Design review of the part built by this model. Coordinates are the model's own, in mm. Face numbers are marked on the shaded views. A direction names the side the tool comes from. Coordinates: 2 decimals unless noted, no trailing zeros. Loops run counter-clockwise (first coordinate to the right, second up) from the corner with the lowest first, then second, coordinate; pieces in that order, holes last. Notation, with made-up numbers: (83.5, 14.25) - (105.5, 14.25) arc R11 cw to (105.5, 34.25) - close; hole circle Ø7 at (19.5, 54). An arc over 180 degrees is marked (long way). Answer in a Markdown table with one row per item. Add a question column.
(1) Clearance check with flat-ended pins moving along their axes: pin 1 (12 mm diameter, centred on x = -8, y = 36.5, fed in from +Z); pin 2 (21 mm diameter, centred on x = 0, z = 0, fed in from -Y); pin 3 (1 mm diameter, centred on x = -13.5, y = 28.5, fed in from +Z); pin 4 (2 mm diameter, centred on y = 15.5, z = -2.5, fed in from +X). State where each tip first meets the part, or that it passes through.
(2) To check wall thickness, follow L1, parallel to Z at x = 0, y = 32; L2, parallel to X at y = 34, z = -16; L3, parallel to Z at x = 0, y = 92. State the ranges of each line that lie inside material, in increasing order. Write a range as [from, to].
(3) For the marked faces 1 and 2, list the 3-axis set-ups (+Z, -Z, +X, -X, +Y, -Y) from which the entire face can be reached by the end or side of a thin tool; tool diameter is ignored.
(4) We need section A-A, the plane z = 0. Write out the cut boundary in (x, y), plus the area to 3 significant figures.
(5) The part is to be moulded in two halves that separate along X. For the marked faces 3 and 4, say which applies: released by +X, released by -X, zero draft, split by the parting line, or undercut.
(6) We need section C-C, the plane y = 79. Write out the cut boundary in (x, z), plus the area to 3 significant figures.
(7) We need section B-B, the plane x = 0. Write out the cut boundary in (y, z).
(8) We need section D-D, the plane y = 35.5. Write out the cut boundary in (x, z), plus the area to 3 significant figures.
Autodesk Inventor part; units mm, degrees
ref_plane "YZ Plane" through (0, 0, 0) normal (1, 0, 0) x (0, 1, 0)
ref_plane "XZ Plane" through (0, 0, 0) normal (0, 1, 0) x (-1, 0, 0)
ref_plane "XY Plane" through (0, 0, 0) normal (0, 0, 1) x (1, 0, 0)
sketch "Sketch1" plane through (0, 0, 0) normal (0, 0, 1) x (1, 0, 0)
  line L0 (0, 0) -> (0, 68.7718)
  line L1 (0, 0) -> (-35.2548, 0) construction
  line L2 (-19.05, 0) -> (-19.05, 50.8)
  line L3 (-19.05, 50.8) -> (-12.7, 76.2)
  line L4 (-12.7, 76.2) -> (-12.7, 127)
  line L5 (-11.05, 127) -> (-11.05, 75.9969)
  line L6 (-11.05, 75.9969) -> (-17.4, 50.5969)
  line L7 (-17.4, 50.5969) -> (-17.4, 0)
  line L8 (-19.05, 0) -> (-17.4, 0)
  line L9 (-12.7, 127) -> (-11.05, 127)
  dimension "d0" = 1.65
  dimension "d1" = 25.4
  dimension "d2" = 50.8
  dimension "d3" = 50.8
  dimension "d4" = 127
  dimension "d5" = 38.1
revolve "Revolution1" add sketch "Sketch1" angle 360 about axis through (0, 0, 0) along (0, 1, 0)
equation "\"d2\" = 0.4 * d4"
equation "\"d3\" = d2"
properties part number "ASME BPE CON RED-38.1-25.4"
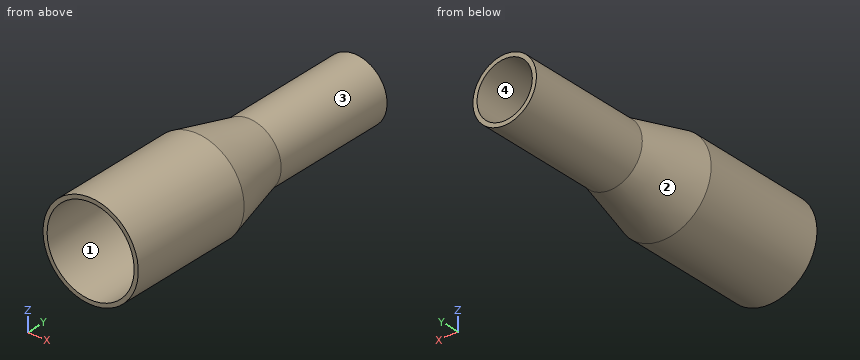
Responses:
| question | item | result |
|---|---|---|
| 1 | pin 1 | stops at z = 18.94 |
| 1 | pin 2 | passes through |
| 1 | pin 3 | stops at z = 13.92 |
| 1 | pin 4 | stops at x = 18.99 |
| 2 | L1 | z = [-19.05, -17.4], [17.4, 19.05] |
| 2 | L2 | x = [-10.34, -6.84], [6.84, 10.34] |
| 2 | L3 | z = [-12.7, -11.05], [11.05, 12.7] |
| 3 | face 1 | -Y |
| 3 | face 2 | +Y |
| 4 | outline | (-19.05, 0) - (-17.4, 0) - (-17.4, 50.6) - (-11.05, 76) - (-11.05, 127) - (-12.7, 127) - (-12.7, 76.2) - (-19.05, 50.8) - close; (11.05, 76) - (17.4, 50.6) - (17.4, 0) - (19.05, 0) - (19.05, 50.8) - (12.7, 76.2) - (12.7, 127) - (11.05, 127) - close |
| 4 | area | 422 mm2 |
| 5 | face 3 | split by the parting line |
| 5 | face 4 | undercut |
| 6 | outline | circle Ø25.4 at (0, 0); hole circle Ø22.1 at (0, 0) |
| 6 | area | 123 mm2 |
| 7 | outline | (0, -19.05) - (50.8, -19.05) - (76.2, -12.7) - (127, -12.7) - (127, -11.05) - (76, -11.05) - (50.6, -17.4) - (0, -17.4) - close; (0, 17.4) - (50.6, 17.4) - (76, 11.05) - (127, 11.05) - (127, 12.7) - (76.2, 12.7) - (50.8, 19.05) - (0, 19.05) - close |
| 8 | outline | circle Ø38.1 at (0, 0); hole circle Ø34.8 at (0, 0) |
| 8 | area | 189 mm2 |
